Geometry: final body of the model. Coordinates: model frame, mm. A direction names the side the tool comes from. Give positions to 0.01 mm unless a question says otherwise; leave off trailing zeros. Loops run counter-clockwise (first coordinate to the right, second up) from the corner with the lowest first, then second, coordinate; pieces in that order, holes last.
from build123d import *

# Parameters (mm, degrees)
ESBO_O1_R                = 2.6
RESSALTO_EXTRUS_O1_DEPTH = 6
FILETE1_R                = 2
FILETE3_R                = 10
FILETE4_R                = 7


with BuildPart() as part:
    # Esboço1 → Ressalto-extrusão1 (new body)
    with BuildSketch(Plane.XY):
        Polygon((-100.5, 95.8), (-22.5, 95.8), (-22.5, -95.8), (-100.5, -95.8), (-100.5, -50.8), (-147.5, -195.8), (-123.706896552, -195.8), (-107.5, -145.8), (-82.5, -127.8), (22.5, -127.8), (22.5, 127.8), (-82.5, 127.8), (-107.5, 145.8), (-123.706896552, 195.8), (-147.5, 195.8), (-100.5, 50.8), align=None)
        with Locations((0, 113.2)):
            Circle(ESBO_O1_R, mode=Mode.SUBTRACT)
        with Locations((0, -113.2)):
            Circle(ESBO_O1_R, mode=Mode.SUBTRACT)
    extrude(amount=RESSALTO_EXTRUS_O1_DEPTH)

    # Filete1
    filete1_edges = [part.edges().sort_by_distance(p)[0] for p in [
        (-100.5, -50.8, 3),
        (-100.5, 50.8, 3),
    ]]
    fillet(filete1_edges, radius=FILETE1_R)

    # Filete3
    filete3_edges = [part.edges().sort_by_distance(p)[0] for p in [
        (-82.5, 127.8, 3),
        (22.5, 127.8, 3),
        (22.5, -127.8, 3),
        (-82.5, -127.8, 3),
        (-107.5, -145.8, 3),
        (-123.706896552, -195.8, 3),
        (-100.5, -95.8, 3),
        (-22.5, -95.8, 3),
        (-22.5, 95.8, 3),
        (-100.5, 95.8, 3),
        (-123.706896552, 195.8, 3),
        (-107.5, 145.8, 3),
    ]]
    fillet(filete3_edges, radius=FILETE3_R)

    # Filete4
    filete4_edges = [part.edges().sort_by_distance(p)[0] for p in [
        (-147.5, -195.8, 3),
        (-147.5, 195.8, 3),
    ]]
    fillet(filete4_edges, radius=FILETE4_R)


solid = part.part
Item 1: Section query A-A on x = -51. Return loops of the section in (y, z), plus the area to 3 significant figures.
Values follow:
outline: (-127.8, 0) - (-95.8, 0) - (-95.8, 6) - (-127.8, 6) - close; (95.8, 0) - (127.8, 0) - (127.8, 6) - (95.8, 6) - close
area: 384 mm2
Item 2: Draft query along Y for faces 1 (the face through (-94.841, 136.686, 2.958)), 2 (the face through (-25.51, 92.95, 3.04)), 3 (the face through (-95.117, -136.884, 2.958)). Return one class per face: +Y half, -Y half, draft (parallel to the pull), parting line (faces both ways), or undercut.
Values follow:
face 1: +Y half
face 2: undercut
face 3: -Y half
Item 3: Section query C-C on y = 11.5. Return loops of the section in (x, z).
Values follow:
outline: (-22.5, 0) - (22.5, 0) - (22.5, 6) - (-22.5, 6) - close
Item 4: Set-up query: faces 4 (the face through (-97.49, -92.95, 3.04)), 5 (the face through (-124.186, -123.874, 2.958)), 6 (the face through (-115.08, -169.18, 2.96)). Return all of +Z, -Z, +X, -X, +Y, -Y with unobstructed straight access to the full face (end or side cutting, diameter ignored); none if empty.
Values follow:
face 4: +Z, -Z
face 5: +Z, -Z, -X
face 6: +Z, -Z, +X, -Y
Item 5: Ray query, probe 1 along Y at (x, z) = (0, 3.5); probe 2 along Y at (x, z) = (-63, 1.95); probe 3 along Y at (x, z) = (-5.5, 4.1). Return the intervals inside material, ascending.
Values follow:
probe 1: y = -127.8 to -115.8, -110.6 to 110.6, 115.8 to 127.8
probe 2: y = -127.8 to -95.8, 95.8 to 127.8
probe 3: y = -127.8 to 127.8
Item 6: Section query B-B on z = 3.7. Give the number of separate pieces and of enclosed holes in the cut face, plus the area to 3 significant figures.
Values follow:
separate pieces: 1
enclosed holes: 2
area: 21,900 mm2
Item 7: Pin query (flat end, axial travel): pin 1 (2 mm diameter, centred on y = 152, z = 1, fed in from +X); pin 2 (1.8 mm diameter, centred on x = -25, z = 3.5, fed in from -Y); pin 3 (3 mm diameter, centred on x = -10.5, z = 4, fed in from +Y); pin 4 (4 mm diameter, centred on x = 0, y = -113.2, fed in from -Z). Return the tip coordinate at first contact, or that it passes through.
Values follow:
pin 1: stops at x = -109.19
pin 2: stops at y = -127.8
pin 3: stops at y = 127.8
pin 4: passes through
